Geometry check sheet. Reference: the model listing, model coordinates, mm. A direction names the side the tool comes from. Coordinates: 2 decimals unless noted, no trailing zeros. Write each loop counter-clockwise with the first axis right and the second up, starting at its lowest first coordinate (ties: lowest second). Pieces come first, ordered by that corner, then holes. Notation, with made-up numbers: (-1.5, 77) -> (50.5, 77) arc R15 cw to (50.5, 94) -> close; hole circle Ø9 at (-18, 40.5). An arc over 180 degrees is marked (long way). One line per question, with ' | ' between items.
```python
from build123d import *

# Parameters (mm, degrees)
SKETCH2_R                = 13.45
BOSS_EXTRUDE1_DEPTH      = 48
CUT_EXTRUDE1_DEPTH       = 10
BOSS_EXTRUDE2_DEPTH      = 13
BOSS_EXTRUDE2_DEPTH_BACK = 2
SKETCH5_W                = 14
SKETCH5_H                = 14
SKETCH5_R                = 4.1


with BuildPart() as part:
    # Sketch2 → Boss-Extrude1 (new body)
    with BuildSketch(Plane(origin=(0, 0, 0), x_dir=(1, 0, 0), z_dir=(0, 1, 0))):
        Polygon((-17.4, -17.4), (17.4, -17.4), (17.4, 0), (58.6, 25.6), (82.6, 25.6), (82.6, 29.6), (58.6, 29.6), (-17.4, 17.4), align=None)
        with Locations(Location((0, 0, 0), (0, 0, 270))):
            Circle(SKETCH2_R, mode=Mode.SUBTRACT)
    boss_extrude1 = extrude(amount=BOSS_EXTRUDE1_DEPTH)

    # Mirror1: Boss-Extrude1 across plane
    add(boss_extrude1.mirror(Plane(origin=(82.6, 0, 0), x_dir=(0, 0, 1), z_dir=(1, 0, 0))))

    # Sketch4 → Cut-Extrude1 (cut)
    with BuildSketch(Plane(origin=(0, 0, -29.6), x_dir=(-1, 0, 0), z_dir=(0, 0, -1))):
        with BuildLine():
            Line((-101.6, 10.3), (-63.6, 10.3))
            ThreePointArc((-63.6, 10.3), (-61.85, 8.55), (-63.6, 6.8))
            Line((-63.6, 6.8), (-101.6, 6.8))
            ThreePointArc((-101.6, 6.8), (-103.35, 8.55), (-101.6, 10.3))
        make_face()
        with BuildLine():
            Line((-101.6, 37.7), (-63.6, 37.7))
            ThreePointArc((-63.6, 37.7), (-61.85, 39.45), (-63.6, 41.2))
            Line((-63.6, 41.2), (-101.6, 41.2))
            ThreePointArc((-101.6, 41.2), (-103.35, 39.45), (-101.6, 37.7))
        make_face()
        with BuildLine():
            Line((-89.6, 12), (-75.6, 12))
            ThreePointArc((-75.6, 12), (-72.064466094, 13.464466094), (-70.6, 17))
            Line((-70.6, 17), (-70.6, 31))
            ThreePointArc((-70.6, 31), (-72.064466094, 34.535533906), (-75.6, 36))
            Line((-75.6, 36), (-89.6, 36))
            ThreePointArc((-89.6, 36), (-93.135533906, 34.535533906), (-94.6, 31))
            Line((-94.6, 31), (-94.6, 17))
            ThreePointArc((-94.6, 17), (-93.135533906, 13.464466094), (-89.6, 12))
        make_face()
    extrude(amount=-CUT_EXTRUDE1_DEPTH, mode=Mode.SUBTRACT)

    # Sketch5 → Boss-Extrude2 (add, two sides: drawn at the far end of the back side and taken through both)
    with BuildSketch(Plane(origin=(0, 0, -29.6), x_dir=(-1, 0, 0), z_dir=(0, 0, -1)).offset(-BOSS_EXTRUDE2_DEPTH_BACK)):
        with Locations((-62.1, 24.09990131)):
            Rectangle(SKETCH5_W, SKETCH5_H)
        with Locations((-62.1, 24.09990131)):
            Circle(SKETCH5_R, mode=Mode.SUBTRACT)
    extrude(amount=BOSS_EXTRUDE2_DEPTH + BOSS_EXTRUDE2_DEPTH_BACK)


solid = part.part
```
(1) Tool access check on faces 4 (the face through (83, 36, -28)), 5 (the face through (66.196, 24.28, -35.96)), 6 (the face through (-17.4, 24, 0)), 7 (the face through (76, 0, -27)), 8 (the face through (37.71, 23.66, -12.62)). Record the directions out of +Z, -Z, +X, -X, +Y, -Y that give a thin tool (end or side, any length) a straight path to the whole face; none if there is none.
Answers below:
face 4: +Z, -Z | face 5: -Z | face 6: +Z, -Z, -X, +Y, -Y | face 7: +Z, -Z, +X, -X, -Y | face 8: +Z, +Y, -Y
(2) Draft check along Z on faces 1 (the face through (127.49, 23.66, -12.62)), 2 (the face through (69.1, 24, -36)), 3 (the face through (-13.13, 23.66, -2.92)). Enter one of: pulls with the +Z half, pulls with the -Z half, needs draft (parallel to the pull), parting line crosses it, or undercut.
Answers below:
face 1: pulls with the +Z half | face 2: needs draft | face 3: undercut
(3) Depth check by flat-ended pin: P1, Ø10, axis at x = 94.5, y = 42, coming from the +Z side; P2, Ø1.5, axis at x = 112, y = 11.5, coming from the -Z side; P3, Ø7, axis at x = 62.5, z = -38.5, coming from the -Y side. Enter the tip coordinate at first touch or a pass-through.
Answers below:
P1: stops at z = -25.6 | P2: stops at z = -28.85 | P3: stops at y = 17.1
(4) Cross-section at C-C (z = 9). Record the cut outline in (x, y).
Answers below:
outline: (-17.4, 0) -> (-10, 0) -> (-10, 48) -> (-17.4, 48) -> close; (10, 0) -> (17.4, 0) -> (17.4, 48) -> (10, 48) -> close; (147.8, 0) -> (155.2, 0) -> (155.2, 48) -> (147.8, 48) -> close; (175.2, 0) -> (182.6, 0) -> (182.6, 48) -> (175.2, 48) -> close
(5) Material ranges on line 1 (X direction, y = 37, z = 0); line 2 (Y direction, x = 62.1, z = -36); line 3 (X direction, y = 37, z = 8), recorded low to high.
Answers below:
line 1: x = -17.4 to -13.45, 13.45 to 17.4, 147.8 to 151.75, 178.65 to 182.6 | line 2: y = 17.1 to 20, 28.2 to 31.1 | line 3: x = -17.4 to -10.81, 10.81 to 17.4, 147.8 to 154.39, 176.01 to 182.6
(6) Cross-section at B-B (x = 165.2). Record the cut outline in (y, z).
Answers below:
outline: (0, -20.19) -> (48, -20.19) -> (48, -13.45) -> (0, -13.45) -> close; (0, 13.45) -> (48, 13.45) -> (48, 17.4) -> (0, 17.4) -> close
(7) Cross-section at D-D (z = -34). Record the cut outline in (x, y).
Answers below:
outline: (55.1, 17.1) -> (69.1, 17.1) -> (69.1, 31.1) -> (55.1, 31.1) -> close; hole circle Ø8.2 at (62.1, 24.1)
(8) Cross-section at A-A (y = 8.55). Record the cut outline in (x, z), plus the area to 3 significant figures.
Answers below:
outline: (-17.4, -17.4) -> (58.6, -29.6) -> (61.85, -29.6) -> (61.85, -25.6) -> (58.6, -25.6) -> (17.4, 0) -> (17.4, 17.4) -> (-17.4, 17.4) -> close; (103.35, -29.6) -> (106.6, -29.6) -> (182.6, -17.4) -> (182.6, 17.4) -> (147.8, 17.4) -> (147.8, 0) -> (106.6, -25.6) -> (103.35, -25.6) -> close; hole circle Ø26.9 at (0, 0); hole circle Ø26.9 at (165.2, 0) | area: 2,620 mm²
